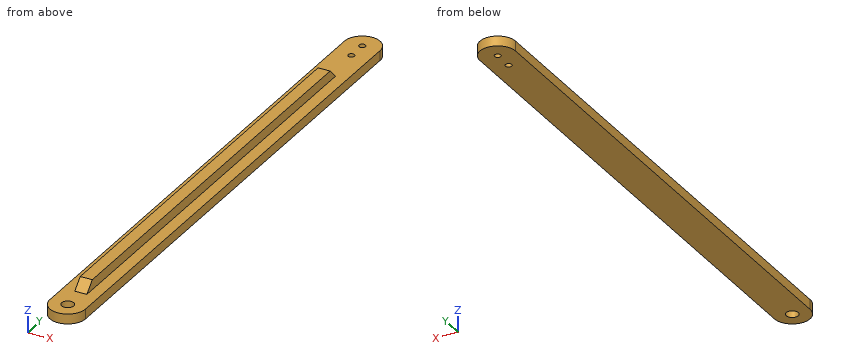
```python
from build123d import *

# Parameters (mm, degrees)
SKETCH1_R           = 3.05
BOSS_EXTRUDE1_DEPTH = 5
SKETCH2_R           = 1.6
CUT_EXTRUDE1_DEPTH  = 10
BOSS_EXTRUDE2_DEPTH = 5
CHAMFER1_SIZE       = 5


with BuildPart() as part:
    # Sketch1 → Boss-Extrude1 (new body)
    with BuildSketch(Plane.XY):
        with BuildLine():
            Line((9, 270), (9, 0))
            ThreePointArc((9, 0), (0, -9), (-9, 0))
            Line((-9, 0), (-9, 270))
            ThreePointArc((-9, 270), (0, 279), (9, 270))
        make_face()
        Circle(SKETCH1_R, mode=Mode.SUBTRACT)
    extrude(amount=BOSS_EXTRUDE1_DEPTH)

    # Sketch2 → Cut-Extrude1 (cut)
    with BuildSketch(Plane.XY.offset(5)):
        with Locations((0, 270)):
            Circle(SKETCH2_R)
        with Locations((0, 260)):
            Circle(SKETCH2_R)
    extrude(amount=-CUT_EXTRUDE1_DEPTH, mode=Mode.SUBTRACT)

    # Sketch3 → Boss-Extrude2 (add)
    with BuildSketch(Plane.XY.offset(5)):
        Polygon((-3.05, 12), (-3.05, 240), (3.05, 240), (3.05, 12), (0, 12), align=None)
    extrude(amount=BOSS_EXTRUDE2_DEPTH)

    # Chamfer1
    chamfer1_edges = [part.edges().sort_by_distance(p)[0] for p in [
        (0, 240, 10),
        (0, 12, 10),
    ]]
    chamfer(chamfer1_edges, length=CHAMFER1_SIZE - 0.0001)  # a hair under: the kernel refuses the full size


solid = part.part
```
Model file for the job. Use its own axes, mm. Give positions to 0.01 mm unless a question says otherwise; leave off trailing zeros. Loops run counter-clockwise (first coordinate to the right, second up) from the corner with the lowest first, then second, coordinate; pieces in that order, holes last. Notation, with made-up numbers: (17.25, 10.5) -> (36.25, 10.5) arc R16 cw to (36.25, 39.5) -> close; hole circle Ø1 at (9, 13). An arc over 180 degrees is marked (long way). Use CSV: the item, a comma, the result in double quotes. Start each with the question number.
1) Flat gauge pins, fed straight in: pin 1 Ø1 at (y, z) = (228.5, 6.5) entering from -X; pin 2 Ø6 at (x, z) = (-4.5, 5.5) entering from +Y; pin 3 Ø1.5 at (x, z) = (-2.5, 6.5) entering from +Y; pin 4 Ø1.9 at (x, y) = (0, 270) entering from -Z. Where does each tip first touch, or does it go through?
2) Slice it at A-A on z = 2.25. Give the cut face in (x, y).
3) Wall check: line 1 (Y direction, x = 0, z = 1.2); line 2 (X direction, y = 260, z = 3.05); line 3 (Z direction, x = 5, y = 207). Give the ranges that are in metal, low to high.
4) Slice it at B-B on y = 197.5. Give the cut face in (x, z), plus the area to 4 significant figures.
5) Slice it at C-C on x = -5.75. Give the cut face in (y, z), plus the area to 3 significant figures.
Computed values:
1,pin 1,"stops at x = -3.05"
1,pin 2,"stops at y = 278.87"
1,pin 3,"stops at y = 239.25"
1,pin 4,"passes through"
2,outline,"(-9, 0) arc R9 ccw to (9, 0) -> (9, 270) arc R9 ccw to (-9, 270) -> close; hole circle Ø6.1 at (0, 0); hole circle Ø3.2 at (0, 260); hole circle Ø3.2 at (0, 270)"
3,line 1,"y = -9 to -3.05, 3.05 to 258.4, 261.6 to 268.4, 271.6 to 279"
3,line 2,"x = -9 to -1.6, 1.6 to 9"
3,line 3,"z = 0 to 5"
4,outline,"(-9, 0) -> (9, 0) -> (9, 5) -> (3.05, 5) -> (3.05, 10) -> (-3.05, 10) -> (-3.05, 5) -> (-9, 5) -> close"
4,area,"120.5 mm^2"
5,outline,"(-6.92, 0) -> (276.92, 0) -> (276.92, 5) -> (-6.92, 5) -> close"
5,area,"1,420 mm^2"
